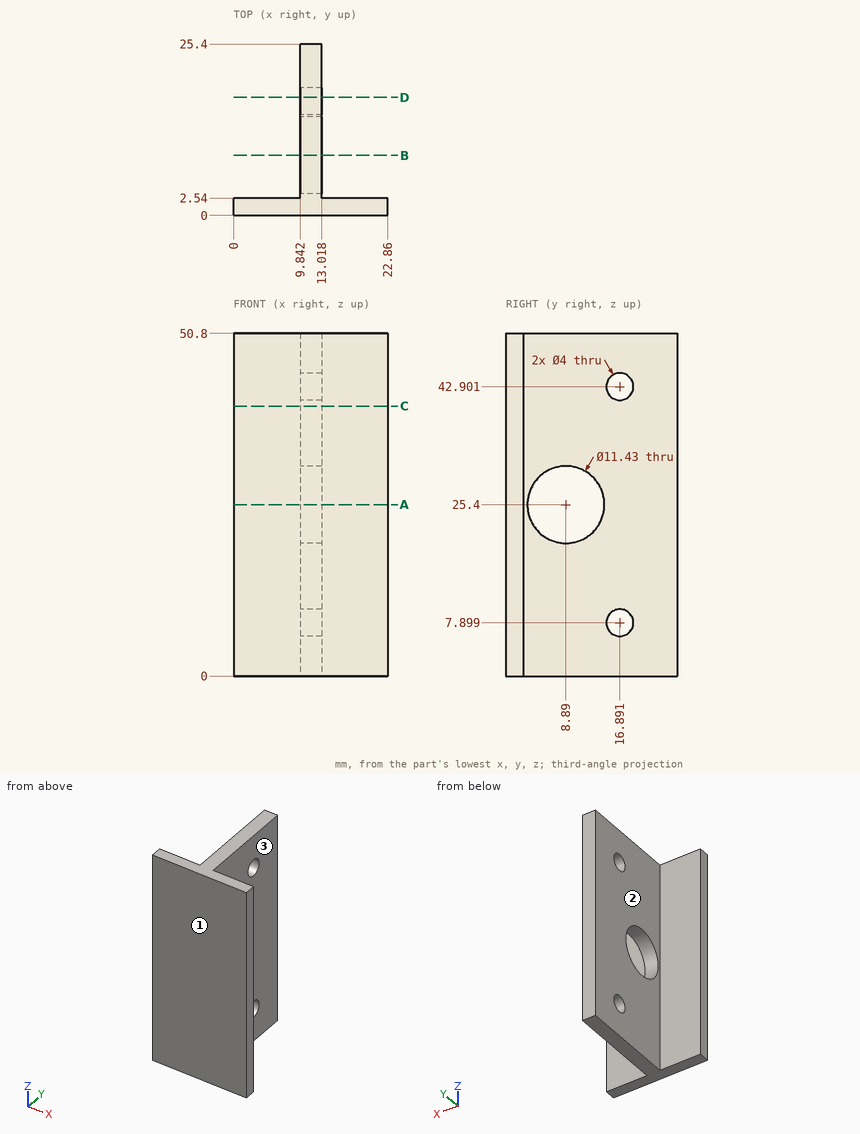
Design review of the part shown in the three views and the two pictorial views. Dimensions are in mm from the part's minimum x, y and z. A direction names the side the tool comes from. Round coordinates to 2 decimals unless told otherwise and drop trailing zeros. Loops run counter-clockwise (first coordinate to the right, second up) from the corner with the lowest first, then second, coordinate; pieces in that order, holes last. Notation, with made-up numbers: (58, 29.25) -> (107, 29.25) arc R17 ccw to (107, 60.25) -> close; hole circle Ø3 at (15, 57.5). An arc over 180 degrees is marked (long way). Use one line per item in the form item = value. Start each with the question number.
Q1. Machinability: for the marked faces 1, 2 and 3, which of the approach directions +Z, -Z, +X, -X, +Y, -Y give a long, thin tool a straight path to every point of the face, cutting with its end or side? Answer none if there is none.
Q2. We need section B-B on y = 8.89. Give the boundary of the cut face in (x, z) (1 decimal).
Q3. We need section D-D on y = 17.5. Give the boundary of the cut face in (x, z) (1 decimal), then the cut area to 3 significant figures.
Q4. Wall thickness on line 1 along Z through (x, y) = (10.25, 15.5) (1 decimal); line 2 along Y through (x, z) = (10.75, 25.4) (1 decimal); line 3 along Y through (x, z) = (21.5, 35): over which ranges is each line inside the solid? List them lowest first. Write a range as [from, to].
Q5. We need section C-C on z = 40. Give the boundary of the cut face in (x, y), then the cut area to 3 significant figures.
Q6. For pin 1 Ø2 at (y, z) = (8.5, 34.5) entering from +X; pin 2 Ø5 at (x, z) = (4, 18) entering from +Y; pin 3 Ø4.5 at (y, z) = (16.89, 7.9) entering from -X, all flat-tipped, find the tip position at first contact; note any pin that passes through.
Q7. We need section A-A on z = 25.4. Give the boundary of the cut face in (x, y) (1 decimal).
Calculated:
q1.face_1 = +Z, -Z, +X, -X, -Y
q1.face_2 = +Z, -Z, -X, +Y
q1.face_3 = +Z, -Z, +X, +Y
q2.outline = (9.8, 0) -> (13, 0) -> (13, 19.7) -> (9.8, 19.7) -> close; (9.8, 31.1) -> (13, 31.1) -> (13, 50.8) -> (9.8, 50.8) -> close
q3.outline = (9.8, 0) -> (13, 0) -> (13, 6) -> (9.8, 6) -> close; (9.8, 9.8) -> (13, 9.8) -> (13, 41) -> (9.8, 41) -> close; (9.8, 44.8) -> (13, 44.8) -> (13, 50.8) -> (9.8, 50.8) -> close
q3.area = 137 mm²
q4.line_1 = [0, 6.5], [9.3, 41.5], [44.3, 50.8]
q4.line_2 = [0, 3.2], [14.6, 25.4]
q4.line_3 = [0, 2.54]
q5.outline = (0, 0) -> (22.86, 0) -> (22.86, 2.54) -> (13.02, 2.54) -> (13.02, 25.4) -> (9.84, 25.4) -> (9.84, 2.54) -> (0, 2.54) -> close
q5.area = 131 mm²
q6.pin_1 = 13.02
q6.pin_2 = 2.54
q6.pin_3 = 9.84
q7.outline = (0, 0) -> (22.9, 0) -> (22.9, 2.5) -> (13, 2.5) -> (13, 3.2) -> (9.8, 3.2) -> (9.8, 2.5) -> (0, 2.5) -> close; (9.8, 14.6) -> (13, 14.6) -> (13, 25.4) -> (9.8, 25.4) -> close
